Input: dimensioned drawing with shaded views. Units: mm. Origin: part minimum x, y, z. Give positions to 0.01 mm unless a question says otherwise; leave off trailing zeros. Write each loop counter-clockwise with the first axis right and the second up, starting at its lowest first coordinate (ties: lowest second). Pieces come first, ordered by that corner, then holes. Notation, with made-up numbers: M 14,-16.5 L 23,-16.5 A25 ccw 23,9.5 Z; hole C 69.5,44 d6. An arc over 180 degrees is marked long. Answer as a JSON object with one key per item and string values.
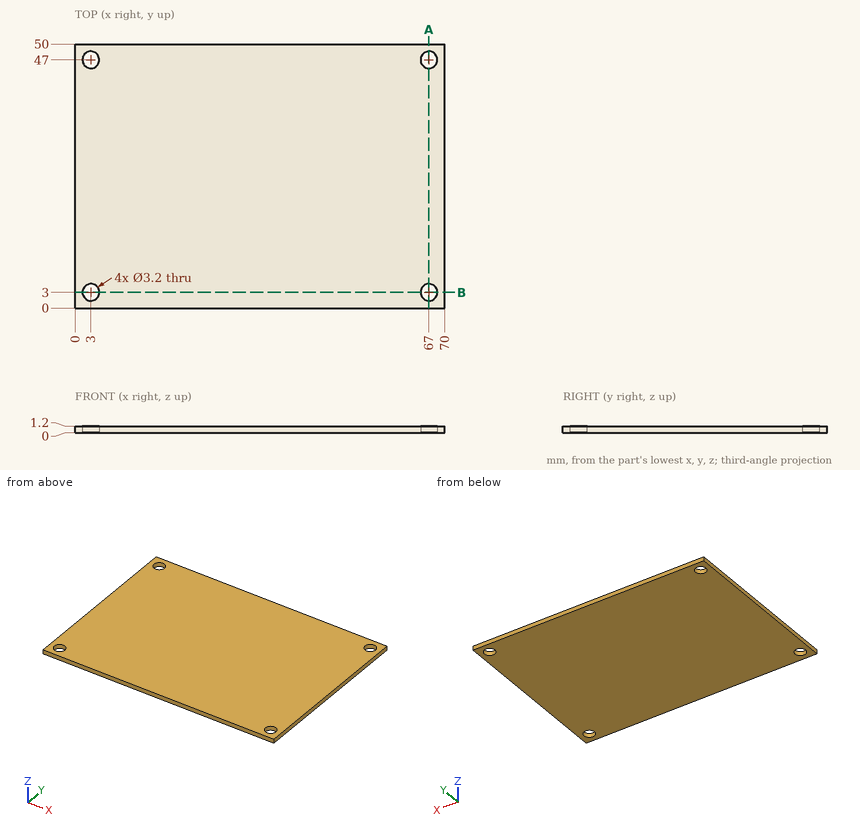
1) Cut plane A-A on x = 67. Return loops of the section in (y, z), and give its area (3 significant figures).
Geometry check:
{"outline": "M 0,0 L 1.4,0 L 1.4,1.2 L 0,1.2 Z; M 4.6,0 L 45.4,0 L 45.4,1.2 L 4.6,1.2 Z; M 48.6,0 L 50,0 L 50,1.2 L 48.6,1.2 Z", "area": "52.3 mm2"}
2) Cut plane B-B on y = 3. Return loops of the section in (x, z), and give its area (3 significant figures).
Geometry check:
{"outline": "M 0,0 L 1.4,0 L 1.4,1.2 L 0,1.2 Z; M 4.6,0 L 65.4,0 L 65.4,1.2 L 4.6,1.2 Z; M 68.6,0 L 70,0 L 70,1.2 L 68.6,1.2 Z", "area": "76.3 mm2"}
3) Contact query for a flat-ended pin moving along its axis: P1, Ø2.5, axis at x = 3, y = 47, coming from the -Z side (3 decimals). Output: stop coordinate, or through.
Geometry check:
{"P1": "passes through"}
4) Line query: line 1 (Y direction, x = 67, z = 0.7). Output: solid intervals per line, ascending. Write a range as from..to.
Geometry check:
{"line 1": "y = 0..1.4, 4.6..45.4, 48.6..50"}
